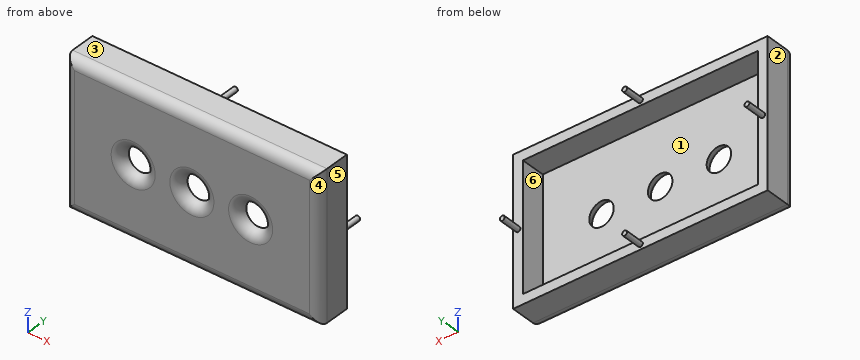
from build123d import *

# Parameters (mm, degrees)
SKETCH1_W           = 66.04
SKETCH1_H           = 38.1
BOSS_EXTRUDE3_DEPTH = 17.78
SKETCH3_W           = 60.96
SKETCH3_H           = 33.02
CUT_EXTRUDE1_DEPTH  = 15.24
SKETCH4_W           = 38.1
SKETCH4_H           = 8.89
CUT_EXTRUDE2_DEPTH  = 66.04
SKETCH5_R           = 0.635
BOSS_EXTRUDE4_DEPTH = 5.08
SKETCH6_R           = 3.175
CUT_EXTRUDE4_DEPTH  = 2.54
FILLET1_R           = 2.54


with BuildPart() as part:
    # Sketch1 → Boss-Extrude3 (new body)
    with BuildSketch(Plane(origin=(0, 0, 0), x_dir=(1, 0, 0), z_dir=(0, 1, 0))):
        with Locations((33.02, 19.05)):
            Rectangle(SKETCH1_W, SKETCH1_H)
    extrude(amount=BOSS_EXTRUDE3_DEPTH)

    # Sketch3 → Cut-Extrude1 (cut)
    with BuildSketch(Plane(origin=(0, 17.78, 0), x_dir=(1, 0, 0), z_dir=(0, 1, 0))):
        with Locations((33.02, 19.05)):
            Rectangle(SKETCH3_W, SKETCH3_H)
    extrude(amount=-CUT_EXTRUDE1_DEPTH, mode=Mode.SUBTRACT)

    # Sketch4 → Cut-Extrude2 (cut)
    with BuildSketch(Plane(origin=(66.04, 0, 0), x_dir=(0, 0, -1), z_dir=(1, 0, 0))):
        with Locations((19.05, 13.335)):
            Rectangle(SKETCH4_W, SKETCH4_H)
    extrude(amount=-CUT_EXTRUDE2_DEPTH, mode=Mode.SUBTRACT)

    # Sketch5 → Boss-Extrude4 (add)
    with BuildSketch(Plane(origin=(0, 8.89, 0), x_dir=(1, 0, 0), z_dir=(0, 1, 0))):
        with Locations(Location((33.02, 36.83, 0), (0, 0, 90))):
            Circle(SKETCH5_R)
        with Locations(Location((33.02, 1.27, 0), (0, 0, 90))):
            Circle(SKETCH5_R)
        with Locations(Location((1.27, 19.05, 0), (0, 0, 90))):
            Circle(SKETCH5_R)
        with Locations(Location((64.77, 19.05, 0), (0, 0, 90))):
            Circle(SKETCH5_R)
    extrude(amount=BOSS_EXTRUDE4_DEPTH)

    # Sketch6 → Cut-Extrude4 (cut)
    with BuildSketch(Plane.XZ):
        with Locations(Location((17.78, -19.05, 0), (0, 0, 270))):
            Circle(SKETCH6_R)
        with Locations(Location((33.02, -19.05, 0), (0, 0, 270))):
            Circle(SKETCH6_R)
        with Locations(Location((48.26, -19.05, 0), (0, 0, 270))):
            Circle(SKETCH6_R)
    extrude(amount=-CUT_EXTRUDE4_DEPTH, mode=Mode.SUBTRACT)

    # Fillet1
    fillet1_edges = [part.edges().sort_by_distance(p)[0] for p in [
        (33.02, 0, -38.1),
        (66.04, 0, -19.05),
        (33.02, 0, 0),
        (0, 0, -19.05),
        (17.78, 0, -15.875),
        (33.02, 0, -15.875),
        (48.26, 0, -15.875),
    ]]
    fillet(fillet1_edges, radius=FILLET1_R - 0.0001)  # a hair under: the kernel refuses the full size


solid = part.part
Check sheet for the modelled part. Datum: model origin and axes. Units: mm. Face numbers are marked on the shaded views. A direction names the side the tool comes from. Round coordinates to 2 decimals unless told otherwise and drop trailing zeros. Loops run counter-clockwise (first coordinate to the right, second up) from the corner with the lowest first, then second, coordinate; pieces in that order, holes last. Notation, with made-up numbers: (-9, 65) -> (26, 65) arc R22 ccw to (26, 80) -> close; hole circle Ø9 at (28, 27). An arc over 180 degrees is marked (long way). Put each result on its own line as item: value. Start each with the question number.
1. Scan lines: probe 1 along X at (y, z) = (2.5, -19.05); probe 2 along Z at (x, y) = (17.78, 2.5); probe 3 along X at (y, z) = (3, -12.5). Record each from-to range of solid material in increasing order.
2. Section check D-D (z = -32.5). Enter the section's corners in (x, y).
3. Gauge pin test, flat end, axial feed: pin 1 (16.5 mm diameter, centred on x = 39.5, z = -24.5, fed in from +Y). Record the tip position at first contact, or that the pin passes through.
4. Access from +Z, -Z, +X, -X, +Y, -Y to the whole of each face (thin tool, end or side, straight path). Record for the marked faces 5 and 6.
5. Section check B-B (y = 4.75). Enter the section's corners in (x, z).
6. Draft check along X on the marked faces 1, 2, 3 and 4. Enter one of: +X half, -X half, draft (parallel to the pull), parting line (faces both ways), or undercut.
Findings:
1. probe 1: x = 0 to 14.6, 20.96 to 29.84, 36.2 to 45.08, 51.44 to 66.04
1. probe 2: z = -38.1 to -22.23, -15.87 to 0
1. probe 3: x = 0 to 2.54, 63.5 to 66.04
2. outline: (0, 2.54) arc R2.54 ccw to (2.54, 0) -> (63.5, 0) arc R2.54 ccw to (66.04, 2.54) -> (66.04, 8.89) -> (63.5, 8.89) -> (63.5, 2.54) -> (2.54, 2.54) -> (2.54, 8.89) -> (0, 8.89) -> close
3. pin 1: stops at y = 2.54
4. face 5: +Z, -Z, +X, +Y, -Y
4. face 6: +Y
5. outline: (0, -38.1) -> (66.04, -38.1) -> (66.04, 0) -> (0, 0) -> close; hole (2.54, -35.56) -> (63.5, -35.56) -> (63.5, -2.54) -> (2.54, -2.54) -> close
6. face 1: undercut
6. face 2: -X half
6. face 3: draft
6. face 4: +X half
